Geometry: final body of the model. Coordinates: model frame, mm. Round coordinates to 2 decimals unless told otherwise and drop trailing zeros. Loops run counter-clockwise (first coordinate to the right, second up) from the corner with the lowest first, then second, coordinate; pieces in that order, holes last. Notation, with made-up numbers: M 71.25,-12.5 L 87.25,-12.5 A12 ccw 87.25,0.5 Z; hole C -35,37.25 d7. An arc over 180 degrees is marked long. Answer as a JSON object with one key per item and string values.
from build123d import *

# Parameters (mm, degrees)
BOSS_EXTRUDE1_DEPTH      = 152.4
BOSS_EXTRUDE1_DEPTH_BACK = 152.4
SKETCH3_W                = 69.85
SKETCH3_H                = 1.1938
SKETCH5_OUTSIDE_W        = 134.39
SKETCH5_OUTSIDE_H        = 369.34
CUT_EXTRUDE2_DEPTH       = 157.355175109


with BuildPart() as part:
    # Sketch3 → Boss-Extrude1 (new, two sides: drawn at the far end of the back side and taken through both)
    with BuildSketch(Plane.XY.offset(-BOSS_EXTRUDE1_DEPTH_BACK)):
        Rectangle(SKETCH3_W, SKETCH3_H)
    extrude(amount=BOSS_EXTRUDE1_DEPTH + BOSS_EXTRUDE1_DEPTH_BACK)

    # Sketch5 outside → Cut-Extrude2 (cut, through all)
    with BuildSketch(Plane.XZ.offset(0.5969)):
        Rectangle(SKETCH5_OUTSIDE_W, SKETCH5_OUTSIDE_H)
        Polygon((-28.575, 152.4), (34.925, 127), (34.925, -127), (-28.575, -152.4), (-34.925, -152.4), (-34.925, 152.4), align=None, mode=Mode.SUBTRACT)
    extrude(amount=-CUT_EXTRUDE2_DEPTH, mode=Mode.SUBTRACT)


solid = part.part
1) Section query C-C (x = -20). Return the cut outline in (y, z), and give its area (3 significant figures).
Results:
{"outline": "M -0.6,-148.97 L 0.6,-148.97 L 0.6,148.97 L -0.6,148.97 Z", "area": "356 mm2"}
2) Section query A-A (y = -0.3). Return the cut outline in (x, z) (3 decimals), and give its area (3 significant figures).
Results:
{"outline": "M -34.925,-152.4 L -28.575,-152.4 L 34.925,-127 L 34.925,127 L -28.575,152.4 L -34.925,152.4 Z", "area": "19,700 mm2"}
3) Section query B-B (x = -9). Return the cut outline in (y, z), and give its area (3 significant figures).
Results:
{"outline": "M -0.6,-144.57 L 0.6,-144.57 L 0.6,144.57 L -0.6,144.57 Z", "area": "345 mm2"}
4) Ray query, line 1 (Z direction, x = -21, y = 0.05); line 2 (Z direction, x = 20.5, y = -0.4). Return the intervals inside material, ascending.
Results:
{"line 1": "-149.37 to 149.37", "line 2": "-132.77 to 132.77"}
